Input: dimensioned drawing with shaded views. Units: mm. Origin: part minimum x, y, z. Give positions to 0.01 mm unless a question says otherwise; leave off trailing zeros. Loops run counter-clockwise (first coordinate to the right, second up) from the corner with the lowest first, then second, coordinate; pieces in that order, holes last.
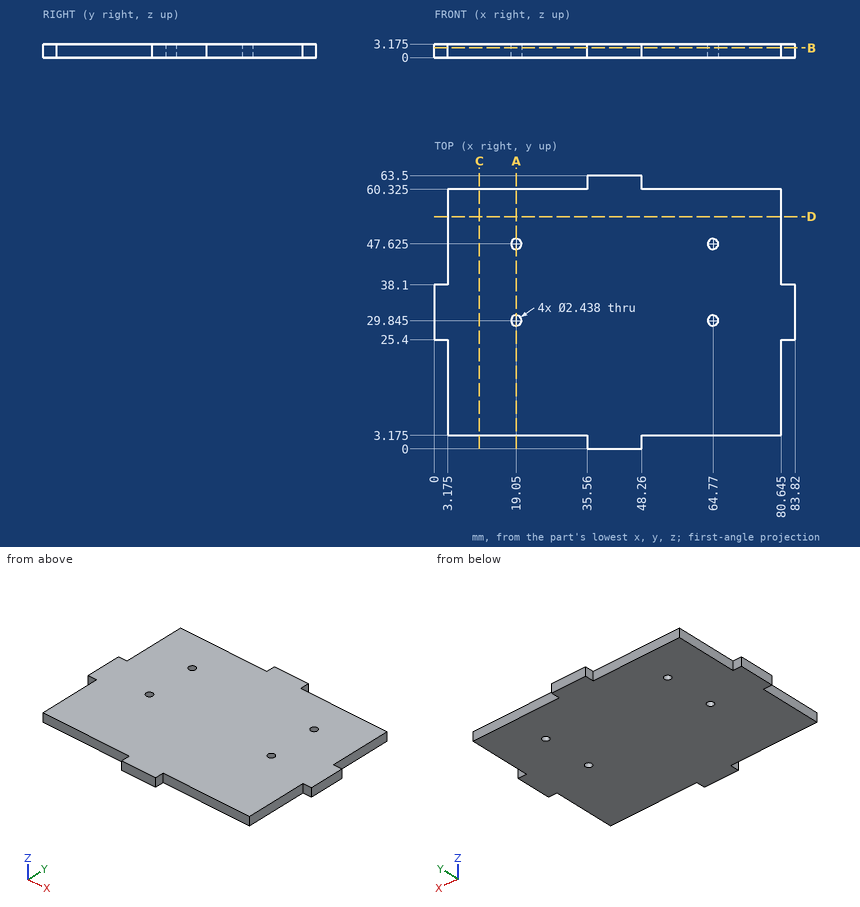
Item 1: Ray query, probe 1 along Y at (x, z) = (64.77, 1.5) (1 decimal); probe 2 along X at (y, z) = (48.5, 1.6) (1 decimal); probe 3 along Y at (x, z) = (77.5, 0.45) (1 decimal). Return the intervals inside material, ascending.
Values follow:
probe 1: y = 3.2 to 28.6, 31.1 to 46.4, 48.8 to 60.3
probe 2: x = 3.2 to 18.2, 19.9 to 63.9, 65.6 to 80.6
probe 3: y = 3.2 to 60.3
Item 2: Section query A-A on x = 19.05. Return loops of the section in (y, z) (1 decimal).
Values follow:
outline: (3.2, 0) - (28.6, 0) - (28.6, 3.2) - (3.2, 3.2) - close; (31.1, 0) - (46.4, 0) - (46.4, 3.2) - (31.1, 3.2) - close; (48.8, 0) - (60.3, 0) - (60.3, 3.2) - (48.8, 3.2) - close
Item 3: Pin query (flat end, axial travel): pin 1 (2 mm diameter, centred on x = 19.05, y = 29.845, fed in from +Z); pin 2 (1 mm diameter, centred on y = 11.5, z = 1.5, fed in from -X) (3 decimals); pin 3 (1.5 mm diameter, centred on x = 69.5, z = 0.5, fed in from +Y) (3 decimals); pin 4 (1 mm diameter, centred on y = 61.5, z = 1.5, fed in from -X). Return the tip coordinate at first contact, or that it passes through.
Values follow:
pin 1: passes through
pin 2: stops at x = 3.175
pin 3: stops at y = 60.325
pin 4: stops at x = 35.56
Item 4: Section query D-D on y = 54. Return loops of the section in (x, z) (1 decimal).
Values follow:
outline: (3.2, 0) - (80.6, 0) - (80.6, 3.2) - (3.2, 3.2) - close
Item 5: Section query C-C on x = 10.5. Return loops of the section in (y, z) (1 decimal).
Values follow:
outline: (3.2, 0) - (60.3, 0) - (60.3, 3.2) - (3.2, 3.2) - close
Item 6: Section query B-B on z = 2.25. Give the number of separate pieces and of enclosed holes in the cut face, plus the area to 3 significant figures.
Values follow:
separate pieces: 1
enclosed holes: 4
area: 4,570 mm2
